```python
from build123d import *

# Parameters (mm, degrees)
F0_W     = 7.7304354078
F0_H     = 21.3139118999
F0_W_2   = 8.8347822961
F0_H_2   = 8.1721762002
F1_DEPTH = 355.6


with BuildPart() as f1:
    # F0 (on Front) → F1 (new body)
    with BuildSketch(Plane.XZ):
        with Locations((0, 14.7430440501)):
            Rectangle(F0_W, F0_H)
        with Locations((-8.282608852, 0)):
            Rectangle(F0_W_2, F0_H_2)
        with Locations((8.282608852, 0)):
            Rectangle(F0_W_2, F0_H_2)
        with Locations((0, -14.7430440501)):
            Rectangle(F0_W, F0_H)
        Rectangle(F0_W, F0_H_2)
    extrude(amount=F1_DEPTH)


solid = f1.part
```
Could you check a few things on this model? Use its own coordinates, in mm. A direction names the side the tool comes from. Give positions to 0.01 mm unless a question says otherwise; leave off trailing zeros. Loops run counter-clockwise (first coordinate to the right, second up) from the corner with the lowest first, then second, coordinate; pieces in that order, holes last. Notation, with made-up numbers: (30.5, 89.5) - (85.5, 89.5) arc R14 ccw to (85.5, 99.5) - close; hole circle Ø2 at (10, 75). An arc over 180 degrees is marked (long way). Use one line per item in the form item = value.
1. On a 3-axis mill with a long thin cutter (end or side, diameter ignored), from which of +Z, -Z, +X, -X, +Y, -Y can I reach the whole of each face in a straight line? I mean faces 1 (the face through (-8, -175, 4.086)), 2 (the face through (8, -175, -4.086)), 3 (the face through (8, -175, 4.086)). Say none if no direction works.
Response values:
face_1 = +Z, -X, +Y, -Y
face_2 = -Z, +X, +Y, -Y
face_3 = +Z, +X, +Y, -Y
2. I want a section at A-A (y = -257.5). Please give me the cut outline in (x, z).
Response values:
outline = (-12.7, -4.09) - (-3.87, -4.09) - (-3.87, -25.4) - (3.87, -25.4) - (3.87, -4.09) - (12.7, -4.09) - (12.7, 4.09) - (3.87, 4.09) - (3.87, 25.4) - (-3.87, 25.4) - (-3.87, 4.09) - (-12.7, 4.09) - close
3. I want a section at C-C (z = -22). Please give me the cut outline in (x, y).
Response values:
outline = (-3.87, -355.6) - (3.87, -355.6) - (3.87, 0) - (-3.87, 0) - close
4. I'm going to push flat-ended pins straight in: pin 1 Ø2 at (y, z) = (-46.5, -6) entering from +X; pin 2 Ø4 at (y, z) = (-195, -12) entering from -X; pin 3 Ø2.5 at (x, y) = (-7, -208) entering from -Z. Where does each tip first touch, or does it pass through?
Response values:
pin_1 = 3.87
pin_2 = -3.87
pin_3 = -4.09
5. I want a section at B-B (x = -7.25). Please give me the cut outline in (y, z), and give its area (3 significant figures).
Response values:
outline = (-355.6, -4.09) - (0, -4.09) - (0, 4.09) - (-355.6, 4.09) - close
area = 2,910 mm²
6. I need wall thicknesses on probe 1 along Z at (x, y) = (-10.5, -194); probe 2 along X at (y, z) = (-337, -5.5). Which ranges of each line are inside material? Lowest first, please.
Response values:
probe_1 = -4.09 to 4.09
probe_2 = -3.87 to 3.87
